For this review, take the finished solid that the model builds, in its own axes (mm). Face numbers are marked on the shaded views. A direction names the side the tool comes from. Coordinates: 2 decimals unless noted, no trailing zeros. Loops run counter-clockwise (first coordinate to the right, second up) from the corner with the lowest first, then second, coordinate; pieces in that order, holes last. Notation, with made-up numbers: M 86.25,-39.5 L 135.25,-39.5 A17 cw 135.25,-20.5 Z; hole C 45,66.25 d9. An arc over 180 degrees is marked long. Write each question's results on one line, items separated by ' | '. Start each with the question number.
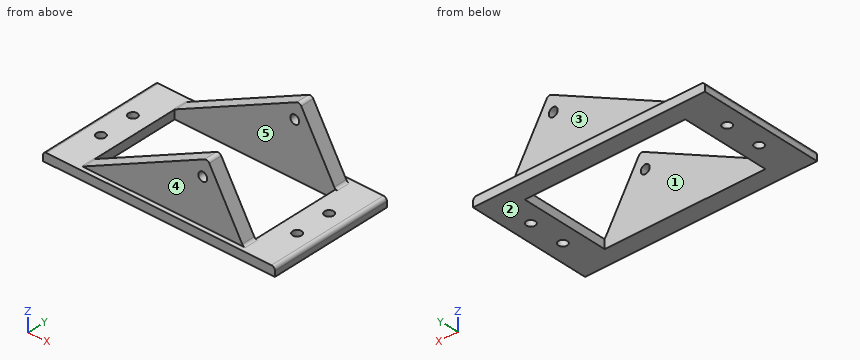
```python
from build123d import *

# Parameters (mm, degrees)
SKETCH1_W           = 165.1
SKETCH1_H           = 88.9
BOSS_EXTRUDE1_DEPTH = 50.8
SKETCH2_R           = 3.175
SKETCH2_W           = 114.3
SKETCH2_H           = 63.5
CUT_EXTRUDE1_DEPTH  = 107.634633211
SKETCH4_W           = 165.1
SKETCH4_H           = 88.9
SKETCH4_W_2         = 114.3
SKETCH4_H_2         = 82.55
CUT_EXTRUDE2_DEPTH  = 44.45
SKETCH5_R           = 3.175
CUT_EXTRUDE4_DEPTH  = 130.398292589
FILLET2_R           = 2.54


with BuildPart() as part:
    # Sketch1 → Boss-Extrude1 (new body)
    with BuildSketch(Plane.XY):
        Rectangle(SKETCH1_W, SKETCH1_H)
    extrude(amount=BOSS_EXTRUDE1_DEPTH)

    # Sketch2 → Cut-Extrude1 (cut, through all)
    with BuildSketch(Plane.XY.offset(50.8)):
        with Locations((-69.85, 12.7)):
            Circle(SKETCH2_R)
        with Locations(Location((-69.85, -12.7, 0), (0, 0, 180))):
            Circle(SKETCH2_R)
        with Locations((69.85, -12.7)):
            Circle(SKETCH2_R)
        with Locations(Location((69.85, 12.7, 0), (0, 0, 180))):
            Circle(SKETCH2_R)
        Rectangle(SKETCH2_W, SKETCH2_H)
    extrude(amount=-CUT_EXTRUDE1_DEPTH, mode=Mode.SUBTRACT)

    # Sketch4 → Cut-Extrude2 (cut)
    with BuildSketch(Plane.XY.offset(50.8)):
        Rectangle(SKETCH4_W, SKETCH4_H)
        Rectangle(SKETCH4_W_2, SKETCH4_H_2, mode=Mode.SUBTRACT)
    extrude(amount=-CUT_EXTRUDE2_DEPTH, mode=Mode.SUBTRACT)

    # Sketch5 → Cut-Extrude4 (cut, through all)
    with BuildSketch(Plane.XZ.offset(41.275)):
        Polygon((-57.15, 6.35), (31.75, 50.8), (-57.15, 50.8), align=None)
        Polygon((31.75, 50.8), (57.15, 6.35), (57.15, 50.8), align=None)
        with Locations((28.286363636, 38.1)):
            Circle(SKETCH5_R)
    extrude(amount=-CUT_EXTRUDE4_DEPTH, mode=Mode.SUBTRACT)

    # Fillet2
    fillet2_edges = [part.edges().sort_by_distance(p)[0] for p in [
        (-57.15, 36.5125, 6.35),
        (-57.15, -36.5125, 6.35),
        (57.15, -36.5125, 6.35),
        (57.15, 36.5125, 6.35),
        (-82.55, 0, 6.35),
        (82.55, 0, 6.35),
        (31.75, -36.5125, 50.8),
        (31.75, 36.5125, 50.8),
    ]]
    fillet(fillet2_edges, radius=FILLET2_R)


solid = part.part
```
Q1. Take a section at C-C, the plane z = 13.5. Give the boundary of the cut face in (x, y) (3 decimals), then the cut area to 3 significant figures.
Q2. Take a section at D-D, the plane y = 12.7. Give the boundary of the cut face in (x, z) (3 decimals), then the cut area to 3 significant figures.
Q3. Take a section at A-A, the plane x = 69.85. Give the boundary of the cut face in (y, z) (3 decimals).
Q4. Insertion check: P1, Ø1, axis at x = 2.5, z = 38, coming from the -Y side (3 decimals); P2, Ø8, axis at x = -16.5, y = 28, coming from the +Z side; P3, Ø10, axis at x = -69.85, y = -12.7, coming from the +Z side; P4, Ø10, axis at x = 28.29, z = 38.1, coming from the -Y side (3 decimals). Each pin has a flat end and moves straight along its axis. Give the tip position at first contact, or say it passes through.
Q5. The part is to be moulded in two halves that separate along X. For the marked faces 1 and 2, say which applies: pulls with the +X half, pulls with the -X half, needs draft (parallel to the pull), parting line crosses it, or undercut.
Q6. For the marked faces 3, 4 and 5, list the 3-axis set-ups (+Z, -Z, +X, -X, +Y, -Y) from which the entire face can be reached by the end or side of a thin tool; tool diameter is ignored.
Q7. To check wall thickness, follow line 1 along Y through (x, z) = (-26, 4.5); line 2 along Y through (x, z) = (16, 14) (3 decimals); line 3 along X through (y, z) = (12, 2). State the ranges of each line that lie inside material, in increasing order.
Q8. Take a section at B-B, the plane y = 38. Give the boundary of the cut face in (x, z) (3 decimals).
Results:
1) outline: M -42.85,-41.275 L 53.064,-41.275 L 53.064,-31.75 L -42.85,-31.75 Z; M -42.85,31.75 L 53.064,31.75 L 53.064,41.275 L -42.85,41.275 Z | area: 1,830 mm^2
2) outline: M -82.55,0 L -73.025,0 L -73.025,6.35 L -80.01,6.35 A2.54 ccw -82.55,3.81 Z; M -66.675,0 L -57.15,0 L -57.15,6.35 L -66.675,6.35 Z; M 57.15,0 L 66.675,0 L 66.675,6.35 L 57.15,6.35 Z; M 73.025,0 L 82.55,0 L 82.55,3.81 A2.54 ccw 80.01,6.35 L 73.025,6.35 Z | area: 239 mm^2
3) outline: M -44.45,0 L -15.875,0 L -15.875,6.35 L -44.45,6.35 Z; M -9.525,0 L 9.525,0 L 9.525,6.35 L -9.525,6.35 Z; M 15.875,0 L 44.45,0 L 44.45,6.35 L 15.875,6.35 Z
4) P1: through | P2: z = 27.37 | P3: z = 6.35 | P4: y = -41.275
5) face 1: undercut | face 2: needs draft
6) face 3: +Z, +X, -X, +Y | face 4: +Z, +X, -X, -Y | face 5: +Z, -Z
7) line 1: -44.45 to -31.75, 31.75 to 44.45 | line 2: -41.275 to -31.75, 31.75 to 41.275 | line 3: -82.55 to -72.95, -66.75 to -57.15, 57.15 to 66.75, 72.95 to 82.55
8) outline: M -82.55,0 L 82.55,0 L 82.55,3.81 A2.54 ccw 80.01,6.35 L 58.624,6.35 A2.54 cw 56.419,7.63 L 32.942,48.714 A2.54 ccw 29.601,49.725 L -56.614,6.618 A2.54 cw -57.75,6.35 L -80.01,6.35 A2.54 ccw -82.55,3.81 Z; hole C 28.286,38.1 d6.35
